from build123d import *

# Parameters (mm, degrees)
F1_DEPTH = 63.5
F2_DEPTH = 25.4
F0_W     = 25.4
F0_H     = 18.5420008242
F0_H_2   = 5.2577991758
F0_H_3   = 4.7752
F3_DEPTH = 25.4


with BuildPart() as f1:
    # F0 (on Front) → F1 (new body, symmetric)
    with BuildSketch(Plane.XZ):
        Polygon((-41.275, 9.525), (-41.275, -9.525), (41.275, -9.525), (41.275, 9.525), (22.7329991758, 9.525), align=None)
    extrude(amount=F1_DEPTH, both=True)

    # F0 (on Front) → F2 (join, symmetric)
    with BuildSketch(Plane.XZ):
        with BuildLine():
            Line((22.7329991758, 9.525), (41.275, 9.525))
            Line((41.275, 9.525), (41.275, 27.0002))
            ThreePointArc((41.275, 27.0002), (45.9246798487, 38.2255201513), (57.15, 42.8752))
            Line((57.15, 42.8752), (60.325, 42.8752))
            Line((60.325, 42.8752), (60.325, 61.4172008242))
            Line((60.325, 61.4172008242), (57.15, 61.4172008242))
            add(Edge.make_bspline(
                [(56.3787146856, 61.4085574833), (56.6358462416, 61.412165765), (56.8929439024, 61.4150481962), (57.15, 61.4172008242)],
                knots=[110.67146519, 110.67146519, 110.67146519, 110.67146519, 111.2667116948, 111.2667116948, 111.2667116948, 111.2667116948], degree=3))
            ThreePointArc((56.3787146856, 61.4085574833), (32.5423256581, 51.0624590215), (22.7329991758, 27.0002))
            Line((22.7329991758, 27.0002), (22.7329991758, 9.525))
        make_face()
    extrude(amount=F2_DEPTH, both=True)

    # F0 (on Front) → F3 (join, symmetric)
    with BuildSketch(Plane.XZ):
        Polygon((-41.275, 9.525), (-41.275, -9.525), (41.275, -9.525), (41.275, 9.525), (22.7329991758, 9.525), align=None)
        with BuildLine():
            add(Edge.make_bspline(
                [(-41.275, 9.525), (-40.4075770381, 34.9754176722), (8.5714183415, 60.7376861335), (56.3787146856, 61.4085574833)],
                knots=[0, 0, 0, 0, 110.67146519, 110.67146519, 110.67146519, 110.67146519], degree=3))
            Line((-41.275, 9.525), (22.7329991758, 9.525))
            Line((22.7329991758, 9.525), (22.7329991758, 27.0002))
            ThreePointArc((22.7329991758, 27.0002), (32.5423256581, 51.0624590215), (56.3787146856, 61.4085574833))
        make_face()
        with BuildLine():
            Line((22.7329991758, 9.525), (41.275, 9.525))
            Line((41.275, 9.525), (41.275, 27.0002))
            ThreePointArc((41.275, 27.0002), (45.9246798487, 38.2255201513), (57.15, 42.8752))
            Line((57.15, 42.8752), (60.325, 42.8752))
            Line((60.325, 42.8752), (60.325, 61.4172008242))
            Line((60.325, 61.4172008242), (57.15, 61.4172008242))
            add(Edge.make_bspline(
                [(56.3787146856, 61.4085574833), (56.6358462416, 61.412165765), (56.8929439024, 61.4150481962), (57.15, 61.4172008242)],
                knots=[110.67146519, 110.67146519, 110.67146519, 110.67146519, 111.2667116948, 111.2667116948, 111.2667116948, 111.2667116948], degree=3))
            ThreePointArc((56.3787146856, 61.4085574833), (32.5423256581, 51.0624590215), (22.7329991758, 27.0002))
            Line((22.7329991758, 27.0002), (22.7329991758, 9.525))
        make_face()
        with Locations((73.025, 52.1462004121)):
            Rectangle(F0_W, F0_H)
        with Locations((73.025, 64.0461004121)):
            Rectangle(F0_W, F0_H_2)
        with Locations((73.025, 40.4876)):
            Rectangle(F0_W, F0_H_3)
        Polygon((85.725, 66.675), (85.725, 61.4172008242), (85.725, 42.8752), (85.725, 38.1), (111.125, 38.1), (111.125, 66.675), align=None)
    extrude(amount=F3_DEPTH, both=True)


solid = f1.part
The model under review builds one solid part; all positions refer to its coordinate system, in mm. A direction names the side the tool comes from. Coordinates: 2 decimals unless noted, no trailing zeros. Loops run counter-clockwise (first coordinate to the right, second up) from the corner with the lowest first, then second, coordinate; pieces in that order, holes last. Notation, with made-up numbers: M 77,20 L 116,20 A17 cw 116,42 Z; hole C 12,6 d11. An arc over 180 degrees is marked long. Put each result on its own line as item: value. Start each with the question number.
Q1. The part is to be moulded in two halves that separate along X. For faces 1 (the flat face through (85, 0, 38.1)), 2 (the flat face through (60.325, 0, 40)), 3 (the flat face through (111.125, 0, 52)), say which applies: +X half, -X half, draft (parallel to the pull), parting line (faces both ways), or undercut.
Q2. Add section A-A (z = 3.5). Write out the cut boundary in (x, y) (3 decimals), and give its area (3 significant figures).
Q3. For faces 4 (the flat face through (1, -45, 9.525)), 5 (the flat face through (60.325, 0, 64)), 6 (the flat face through (34, 25.4, 39)), 7 (the cylindrical face through (45.8, -0.4, 38.1)), 8 (the flat face through (41.275, -1, 4)), list the 3-axis set-ups (+Z, -Z, +X, -X, +Y, -Y) from which the entire face can be reached by the end or side of a thin tool; tool diameter is ignored.
Q4. Wall thickness on line 1 (Y direction, x = 101.5, z = 41.5); line 2 (Z direction, x = 64, y = -11.5) (3 decimals); line 3 (Z direction, x = 30.5, y = -40) (3 decimals): over which ranges is each line inside the solid? List them lowest first.
Q5. Add section B-B (x = 97). Write out the cut boundary in (y, z) (3 decimals).
Q6. Clearance check with flat-ended pins moving along their axes: pin 1 (11 mm diameter, centred on y = 1, z = 12, fed in from +X) (3 decimals); pin 2 (4 mm diameter, centred on x = 36.5, y = -25.5, fed in from +Z); pin 3 (2.5 mm diameter, centred on y = 11.5, z = 63, fed in from -X) (3 decimals). State where each tip first meets the part, or that it passes through.
Answers:
1. face 1: draft
1. face 2: undercut
1. face 3: +X half
2. outline: M -41.275,-63.5 L 41.275,-63.5 L 41.275,63.5 L -41.275,63.5 Z
2. area: 10,500 mm^2
3. face 4: +Z, +X, -X, -Y
3. face 5: +Z, -X, +Y, -Y
3. face 6: +Z, +X, -X, +Y
3. face 7: -Z, +Y, -Y
3. face 8: -Z, +X, +Y, -Y
4. line 1: y = -25.4 to 25.4
4. line 2: z = 38.1 to 66.675
4. line 3: z = -9.525 to 9.525
5. outline: M -25.4,38.1 L 25.4,38.1 L 25.4,66.675 L -25.4,66.675 Z
6. pin 1: stops at x = 41.275
6. pin 2: stops at z = 60.03
6. pin 3: stops at x = 60.325
